```python
from build123d import *

# Parameters (mm, degrees)
F0_W     = 50
F0_H     = 50
F2_R     = 25
F3_DEPTH = 150
F4_DEPTH = 125


with BuildPart() as f1:
    # F0 (on Right) → F1 (revolve)
    with BuildSketch(Plane.YZ):
        with Locations((-325, 25)):
            Rectangle(F0_W, F0_H)
        with BuildLine():
            Line((-300, 0), (0, 0))
            Line((0, 0), (300, 0))
            Line((300, 0), (300, 50))
            ThreePointArc((300, 50), (285.355339, 85.355339), (250, 100))
            Line((250, 100), (-250, 100))
            ThreePointArc((-250, 100), (-285.355339, 85.355339), (-300, 50))
            Line((-300, 50), (-300, 0))
        make_face()
        with Locations((325, 25)):
            Rectangle(F0_W, F0_H)
    revolve(axis=Axis((0, 79.503536, 0), (0, 1, 0)))

    # F2 (on Top) → F3 (join)
    with BuildSketch(Plane.XY):
        with Locations((0, 200)):
            Circle(F2_R)
    extrude(amount=F3_DEPTH)

    # F2 (on Top) → F4 (join)
    with BuildSketch(Plane.XY):
        with Locations((0, -200)):
            Circle(F2_R)
    extrude(amount=-F4_DEPTH)


solid = f1.part
```
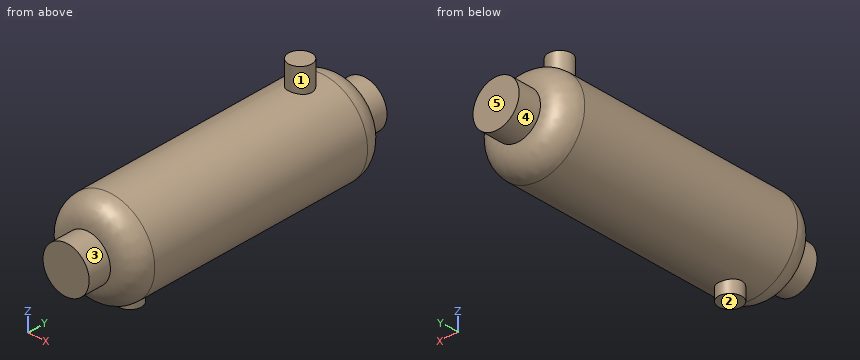
For this review, take the finished solid that the model builds, in its own axes (mm). Face numbers are marked on the shaded views. A direction names the side the tool comes from. Give positions to 0.01 mm unless a question says otherwise; leave off trailing zeros. Write each loop counter-clockwise with the first axis right and the second up, starting at its lowest first coordinate (ties: lowest second). Pieces come first, ordered by that corner, then holes. Notation, with made-up numbers: M 81.25,65.25 L 125.25,65.25 A21 cw 125.25,102.25 Z; hole C -35,-38 d5. An arc over 180 degrees is marked long. Answer as a JSON object with one key per item and string values. Group by question number.
Item 1: Tool access review of the marked faces 1, 2, 3, 4 and 5: name each direction out of +Z, -Z, +X, -X, +Y, -Y from which nothing blocks a thin tool from reaching the whole face with its end or side.
Item 2: Consider section A-A on y = 43. Write out the cut boundary in (x, z).
Item 3: Consider section B-B on y = -200. Write out the cut boundary in (x, z), plus the area to 3 significant figures.
Item 4: For pin 1 Ø3 at (y, z) = (192, 40) entering from +X; pin 2 Ø4 at (x, y) = (27.5, -187.5) entering from +Z; pin 3 Ø12 at (y, z) = (-46.5, 98.5) entering from +X; pin 4 Ø12 at (x, z) = (35.5, 117) entering from -Y, all flat-tipped, find the tip position at first contact; note any pin that passes through.
Item 5: For probe 1 along Z at (x, y) = (24.5, 215); probe 2 along Y at (x, z) = (2, 126.5); probe 3 along Z at (x, y) = (-0.5, -216.5), list the stretches that pass through material, from the lowest coordinate up. Write a range as [from, to].
Check result:
{
 "1": {"face 1": "+Z", "face 2": "-Z, +X, -X, +Y, -Y", "face 3": "-Y", "face 4": "+Y", "face 5": "+Z, -Z, +X, -X, +Y"},
 "2": {"outline": "C 0,0 d200"},
 "3": {"outline": "M -25,-125 L 25,-125 L 25,-96.82 A100 ccw long -25,-96.82 Z", "area": "32,700 mm^2"},
 "4": {"pin 1": "stops at x = 92.29", "pin 2": "stops at z = 96.69", "pin 3": "stops at x = 38", "pin 4": "passes through"},
 "5": {"probe 1": "z = [-96.95, 96.95]", "probe 2": "y = [175.08, 224.92]", "probe 3": "z = [-125, 100]"}
}
